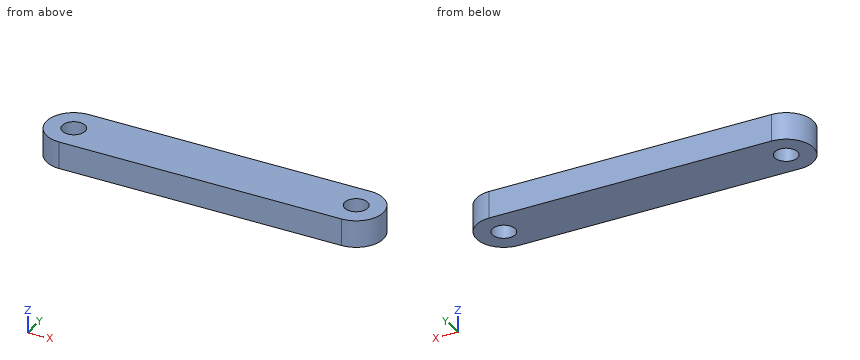
Autodesk Inventor part; units mm, degrees
ref_plane "YZ Plane" through (0, 0, 0) normal (1, 0, 0) x (0, 1, 0)
ref_plane "XZ Plane" through (0, 0, 0) normal (0, 1, 0) x (-1, 0, 0)
ref_plane "XY Plane" through (0, 0, 0) normal (0, 0, 1) x (1, 0, 0)
sketch "Sketch1" plane through (0, 0, 0) normal (0, 0, 1) x (1, 0, 0)
  line L0 (-26, 0) -> (26, 0) construction
  line L1 (-26, -5) -> (26, -5)
  line L2 (26, 5) -> (-26, 5)
  arc A0 (-26, 5) -> (-26, -5) centre (-26, 0) ccw
  arc A1 (26, -5) -> (26, 5) centre (26, 0) ccw
  circle A2 centre (-26, 0) radius 2.1
  circle A3 centre (26, 0) radius 2.1
  point P0 (0, 0)
  point P1 (0, 0)
  point P2 (0, -1.8466)
  point P3 (0, 1.8466)
  dimension "d0" = 10
  dimension "d1" = 52
  dimension "d2" = 4.2
  dimension "d3" = 4.2
extrude "Extrusion1" add sketch "Sketch1" along normal blind 5
equation "\"d2\" = d3"
properties part number "lower-tipper-link"
The listing builds one solid part. Answer for the finished solid, in the listing's coordinates (mm). Give positions to 0.01 mm unless a question says otherwise; leave off trailing zeros. Order: outer loops, then holes, each group sorted by start corner. A loop starts at its lowest first (then second) coordinate and runs counter-clockwise, first axis right, second up. Notation, with made-up numbers: (58, 72) -> (106, 72) arc R13 cw to (106, 94) -> close; hole circle Ø2 at (18.5, 53.5). An arc over 180 degrees is marked (long way). Answer as a JSON object with one key per item and string values. Group by question number.
Item 1: The part is cut by section C-C on y = -3. Write down the section's boundary in (x, z).
Item 2: The part is cut by section A-A on y = 0. Write down the section's boundary in (x, z).
Item 3: Flat-ended cylindrical pins translate along their axes: pin 1 (6 mm diameter, centred on x = 16.5, y = -3.5, fed in from -Z); pin 2 (1 mm diameter, centred on y = -1, z = 2, fed in from -X); pin 3 (2 mm diameter, centred on y = -3.5, z = 3, fed in from -X). Find the tip coordinate at first contact, or state that the pin passes through.
Item 4: Consider L1, parallel to Y at x = 26, z = 3.65; L2, parallel to X at y = 1.25, z = 4.05; L3, parallel to X at y = -0.5, z = 1.15. Determine where each line is inside the solid, lowest interval first. Write a range as from..to.
Item 5: The part is cut by section B-B on z = 2.8. Write down the section's boundary in (x, y), and give its area (3 significant figures).
Result set:
{
 "1": {"outline": "(-30, 0) -> (30, 0) -> (30, 5) -> (-30, 5) -> close"},
 "2": {"outline": "(-31, 0) -> (-28.1, 0) -> (-28.1, 5) -> (-31, 5) -> close; (-23.9, 0) -> (23.9, 0) -> (23.9, 5) -> (-23.9, 5) -> close; (28.1, 0) -> (31, 0) -> (31, 5) -> (28.1, 5) -> close"},
 "3": {"pin 1": "z = 0", "pin 2": "x = -30.97", "pin 3": "x = -30.33"},
 "4": {"L1": "-5..-2.1, 2.1..5", "L2": "-30.84..-27.69, -24.31..24.31, 27.69..30.84", "L3": "-30.97..-28.04, -23.96..23.96, 28.04..30.97"},
 "5": {"outline": "(-26, -5) -> (26, -5) arc R5 ccw to (26, 5) -> (-26, 5) arc R5 ccw to start; hole circle Ø4.2 at (-26, 0); hole circle Ø4.2 at (26, 0)", "area": "571 mm²"}
}
